from build123d import *

# Parameters (mm, degrees)
SKETCH1_W                  = 135.38
SKETCH1_H                  = 172.035
SKETCH1_R                  = 3.2639
SKETCH1_R_2                = 1.4732
BASE_FLANGE1_DEPTH         = 1.6002
SKETCHED_BEND1_OUTLINE_W   = 135.38
SKETCHED_BEND1_OUTLINE_H   = 1.6002
SKETCHED_BEND1_DEPTH       = 129.239310973
SKETCHED_START             = 148.1082001
SKETCHED_BEND1_2_OUTLINE_W = 135.38
SKETCHED_BEND1_2_OUTLINE_H = 1.6002
SKETCHED_BEND1_2_DEPTH     = 23.9267999
SKETCHED_START_2           = 131.860207433
SKETCHED_BEND1_3_OUTLINE_W = 135.38
SKETCHED_BEND1_3_OUTLINE_H = 1.6002
SKETCHED_BEND1_3_DEPTH     = 13.301592467
SKETCHED_START_3           = 130.391703893
SKETCHED_BEND1_4_OUTLINE_W = 135.38
SKETCHED_BEND1_4_OUTLINE_H = 88.066185133
SKETCHED_BEND1_4_OUTLINE_R = 3.2639
SKETCHED_BEND1_4_DEPTH     = 0.14770354
SKETCHED_START_4           = 128.939207433
SKETCHED_BEND1_5_OUTLINE_W = 135.38
SKETCHED_BEND1_5_OUTLINE_H = 88.066185133
SKETCHED_BEND1_5_OUTLINE_R = 3.2639
SKETCHED_BEND1_5_DEPTH     = 2.921
SKETCHED_START_5           = 129.239310973
SKETCHED_BEND1_6_OUTLINE_W = 135.38
SKETCHED_BEND1_6_OUTLINE_H = 1.6002
SKETCHED_BEND1_6_DEPTH     = 18.868889127
SKETCHED_BEND1_7_DEPTH     = 135.38
SKETCHED_START_6           = 87
SKETCHED_BEND1_8_OUTLINE_R = 1.4732
SKETCHED_BEND1_8_DEPTH     = 4


with BuildPart() as part:
    # Base-Flange1: sheet metal written as solids
    # Sketch1 → Base-Flange1 (new body)
    with BuildSketch(Plane(origin=(0, 0, 0), x_dir=(1, 0, 0), z_dir=(0, 1, 0))):
        with Locations((67.69, -86.0175)):
            Rectangle(SKETCH1_W, SKETCH1_H)
        with Locations(Location((67.69, -73.3175, 0), (0, 0, 270))):
            Circle(SKETCH1_R, mode=Mode.SUBTRACT)
        with Locations(Location((67.69, -98.7175, 0), (0, 0, 270))):
            Circle(SKETCH1_R, mode=Mode.SUBTRACT)
        with Locations(Location((54.99, -86.0175, 0), (0, 0, 270))):
            Circle(SKETCH1_R, mode=Mode.SUBTRACT)
        with Locations(Location((80.39, -86.0175, 0), (0, 0, 270))):
            Circle(SKETCH1_R, mode=Mode.SUBTRACT)
        with Locations(Location((38.1, -25.4, 0), (0, 0, 270))):
            Circle(SKETCH1_R_2, mode=Mode.SUBTRACT)
        with Locations(Location((97.28, -25.4, 0), (0, 0, 270))):
            Circle(SKETCH1_R_2, mode=Mode.SUBTRACT)
        with Locations(Location((97.28, -146.635, 0), (0, 0, 90))):
            Circle(SKETCH1_R_2, mode=Mode.SUBTRACT)
        with Locations(Location((38.1, -146.635, 0), (0, 0, 90))):
            Circle(SKETCH1_R_2, mode=Mode.SUBTRACT)
        with Locations(Location((67.69, -25.4, 0), (0, 0, 270))):
            Circle(SKETCH1_R_2, mode=Mode.SUBTRACT)
        with Locations(Location((67.69, -146.635, 0), (0, 0, 270))):
            Circle(SKETCH1_R_2, mode=Mode.SUBTRACT)
    extrude(amount=-BASE_FLANGE1_DEPTH)

    # Sketched Bend1: read off the stored shape, not the designer's step
    # Sketched Bend1 outline → Sketched Bend1 (cut)
    with BuildSketch(Plane.XY):
        with Locations((67.69, -0.8001)):
            Rectangle(SKETCHED_BEND1_OUTLINE_W, SKETCHED_BEND1_OUTLINE_H)
    extrude(amount=SKETCHED_BEND1_DEPTH, mode=Mode.SUBTRACT)

    # Sketched Bend1 4 outline → Sketched Bend1 4 (add)
    with BuildSketch(Plane.XY.offset(SKETCHED_START_3)):
        with Locations((67.69, 44.033092567)):
            Rectangle(SKETCHED_BEND1_4_OUTLINE_W, SKETCHED_BEND1_4_OUTLINE_H)
        with Locations((67.69, 31.333092567)):
            Circle(SKETCHED_BEND1_4_OUTLINE_R, mode=Mode.SUBTRACT)
        with Locations((54.99, 44.033092567)):
            Circle(SKETCHED_BEND1_4_OUTLINE_R, mode=Mode.SUBTRACT)
        with Locations((80.39, 44.033092567)):
            Circle(SKETCHED_BEND1_4_OUTLINE_R, mode=Mode.SUBTRACT)
        with Locations((67.69, 56.733092567)):
            Circle(SKETCHED_BEND1_4_OUTLINE_R, mode=Mode.SUBTRACT)
    extrude(amount=SKETCHED_BEND1_4_DEPTH)



with BuildPart() as body_2:
    # Sketched Bend1 2 outline → Sketched Bend1 2 (new body)
    with BuildSketch(Plane.XY.offset(SKETCHED_START)):
        with Locations((67.69, 88.866285133)):
            Rectangle(SKETCHED_BEND1_2_OUTLINE_W, SKETCHED_BEND1_2_OUTLINE_H)
    extrude(amount=SKETCHED_BEND1_2_DEPTH)


with BuildPart() as body_3:
    # Sketched Bend1 3 outline → Sketched Bend1 3 (new body)
    with BuildSketch(Plane.XY.offset(SKETCHED_START_2)):
        with Locations((67.69, 88.866285133)):
            Rectangle(SKETCHED_BEND1_3_OUTLINE_W, SKETCHED_BEND1_3_OUTLINE_H)
    extrude(amount=SKETCHED_BEND1_3_DEPTH)


with BuildPart() as part_1:
    add(part.part)

    add(body_3.part)  # Sketched Bend1 5 merges body 3
    # Sketched Bend1 5 outline → Sketched Bend1 5 (add)
    with BuildSketch(Plane.XY.offset(SKETCHED_START_4)):
        with Locations((67.69, 44.033092567)):
            Rectangle(SKETCHED_BEND1_5_OUTLINE_W, SKETCHED_BEND1_5_OUTLINE_H)
        with Locations((67.69, 31.333092567)):
            Circle(SKETCHED_BEND1_5_OUTLINE_R, mode=Mode.SUBTRACT)
        with Locations((54.99, 44.033092567)):
            Circle(SKETCHED_BEND1_5_OUTLINE_R, mode=Mode.SUBTRACT)
        with Locations((80.39, 44.033092567)):
            Circle(SKETCHED_BEND1_5_OUTLINE_R, mode=Mode.SUBTRACT)
        with Locations((67.69, 56.733092567)):
            Circle(SKETCHED_BEND1_5_OUTLINE_R, mode=Mode.SUBTRACT)
    extrude(amount=SKETCHED_BEND1_5_DEPTH)


    add(body_2.part)  # Sketched Bend1 6 merges body 2
    # Sketched Bend1 6 outline → Sketched Bend1 6 (add)
    with BuildSketch(Plane.XY.offset(SKETCHED_START_5)):
        with Locations((67.69, 88.866285133)):
            Rectangle(SKETCHED_BEND1_6_OUTLINE_W, SKETCHED_BEND1_6_OUTLINE_H)
    extrude(amount=SKETCHED_BEND1_6_DEPTH)

    # Sketched Bend1 7 outline → Sketched Bend1 7 (cut)
    with BuildSketch(Plane.YZ):
        with BuildLine():
            Line((1.3208, 130.539407433), (86.745385133, 130.539407433))
            ThreePointArc((86.745385133, 130.539407433), (87.67933177, 130.926260797), (88.066185133, 131.860207433))
            Line((88.066185133, 131.860207433), (0, 131.860207433))
            ThreePointArc((0, 131.860207433), (0.386853363, 130.926260797), (1.3208, 130.539407433))
        make_face()
        with BuildLine():
            Line((0, 128.939207433), (1.3208, 128.939207433))
            ThreePointArc((1.3208, 128.939207433), (-0.744658907, 129.794748526), (-1.6002, 131.860207433))
            Line((-1.6002, 131.860207433), (-1.6002, 129.239310973))
            Line((-1.6002, 129.239310973), (0, 129.239310973))
            Line((0, 129.239310973), (0, 128.939207433))
        make_face()
        with BuildLine():
            ThreePointArc((89.666385133, 131.860207433), (88.810844041, 129.794748526), (86.745385133, 128.939207433))
            Line((86.745385133, 128.939207433), (88.066185133, 128.939207433))
            Line((88.066185133, 128.939207433), (88.066185133, 129.239310973))
            Line((88.066185133, 129.239310973), (89.666385133, 129.239310973))
            Line((89.666385133, 129.239310973), (89.666385133, 131.860207433))
        make_face()
    extrude(amount=SKETCHED_BEND1_7_DEPTH, mode=Mode.SUBTRACT)

    # Sketched Bend1 8 outline → Sketched Bend1 8 (cut)
    with BuildSketch(Plane(origin=(0, 0, 0), x_dir=(1, 0, 0), z_dir=(0, 1, 0)).offset(SKETCHED_START_6)):
        with Locations((67.69, -146.635)):
            Circle(SKETCHED_BEND1_8_OUTLINE_R)
        with Locations((97.28, -146.635)):
            Circle(SKETCHED_BEND1_8_OUTLINE_R)
        with Locations((38.1, -146.635)):
            Circle(SKETCHED_BEND1_8_OUTLINE_R)
    extrude(amount=SKETCHED_BEND1_8_DEPTH, mode=Mode.SUBTRACT)


solid = part_1.part
Can you work these out from the model? Positions are in its coordinate system, mm. A direction names the side the tool comes from. Give positions to 0.01 mm unless a question says otherwise; leave off trailing zeros. Loops run counter-clockwise (first coordinate to the right, second up) from the corner with the lowest first, then second, coordinate; pieces in that order, holes last. Notation, with made-up numbers: (-15.75, 75.25) - (21.25, 75.25) arc R26 ccw to (21.25, 90.25) - close; hole circle Ø11 at (-9.75, 87). An arc over 180 degrees is marked (long way). Answer as a JSON object with one key per item and string values.
Q1. Imagine slicing it at A-A on x = 80.39. Write out the boundary of the cut face in (y, z) (3 decimals).
Geometry says:
{"outline": "(-1.6, 131.86) arc R2.921 ccw to (1.321, 128.939) - (40.769, 128.939) - (40.769, 130.539) - (1.321, 130.539) arc R1.321 cw to (0, 131.86) - (0, 172.035) - (-1.6, 172.035) - close; (47.297, 128.939) - (86.745, 128.939) arc R2.921 ccw to (89.666, 131.86) - (89.666, 172.035) - (88.066, 172.035) - (88.066, 131.86) arc R1.321 cw to (86.745, 130.539) - (47.297, 130.539) - close"}
Q2. If I drill on L1, parallel to Y at x = 117.5, z = 155; L2, parallel to Y at x = 67, z = 130; L3, parallel to Z at x = 45.5, y = 28, over which ranges is the centre line in solid material (lowest first)?
Geometry says:
{"L1": "-1.6 to 0, 88.07 to 89.67", "L2": "-0.93 to 28.14, 34.52 to 53.54, 59.92 to 89", "L3": "128.94 to 130.54"}
Q3. Will these pins go through, and if not, where does the flat tip stop? P1, Ø2.5, axis at x = 67.69, z = 146.635, coming from the -Y side; P2, Ø1.5, axis at x = 112, y = 75, coming from the +Z side.
Geometry says:
{"P1": "through", "P2": "z = 130.54"}
Q4. Imagine slicing it at B-B on x = 38.1. Write out the boundary of the cut face in (y, z) (3 decimals), plus the area to 3 significant figures.
Geometry says:
{"outline": "(-1.6, 131.86) arc R2.921 ccw to (1.321, 128.939) - (86.745, 128.939) arc R2.921 ccw to (89.666, 131.86) - (89.666, 145.162) - (88.066, 145.162) - (88.066, 131.86) arc R1.321 cw to (86.745, 130.539) - (1.321, 130.539) arc R1.321 cw to (0, 131.86) - (0, 145.162) - (-1.6, 145.162) - close; (-1.6, 148.108) - (0, 148.108) - (0, 172.035) - (-1.6, 172.035) - close; (88.066, 148.108) - (89.666, 148.108) - (89.666, 172.035) - (88.066, 172.035) - close", "area": "267 mm²"}
Q5. Which directions (+Z, -Z, +X, -X, +Y, -Y) give clear straight access to the entire face, cutting with the end or side of a thin tool? Please do faces 4 (the flat face through (67, 88.066, 152)), 5 (the flat face through (67, 89.666, 152)).
Geometry says:
{"face 4": "+Z, +X, -X", "face 5": "+Z, -Z, +X, -X, +Y"}
Q6. If we mould it in two halves opening along X, with no side actions, what happens to faces 1 (the cylindrical face through (37.66, -0.79, 145.23)), 2 (the flat face through (0, 24, 130)), 3 (the cylindrical face through (66.74, -0.72, 129.77))? For each: pulls with the +X half, pulls with the -X half, needs draft (parallel to the pull), parting line crosses it, or undercut.
Geometry says:
{"face 1": "undercut", "face 2": "pulls with the -X half", "face 3": "needs draft"}
Q7. Imagine slicing it at D-D on x = 9. Write out the boundary of the cut face in (y, z) (3 decimals).
Geometry says:
{"outline": "(-1.6, 131.86) arc R2.921 ccw to (1.321, 128.939) - (86.745, 128.939) arc R2.921 ccw to (89.666, 131.86) - (89.666, 172.035) - (88.066, 172.035) - (88.066, 131.86) arc R1.321 cw to (86.745, 130.539) - (1.321, 130.539) arc R1.321 cw to (0, 131.86) - (0, 172.035) - (-1.6, 172.035) - close"}
Q8. Imagine slicing it at C-C on z = 141.5. Write out the boundary of the cut face in (x, y).
Geometry says:
{"outline": "(0, -1.6) - (135.38, -1.6) - (135.38, 0) - (0, 0) - close; (0, 88.07) - (135.38, 88.07) - (135.38, 89.67) - (0, 89.67) - close"}
